The model under review builds one solid part; all positions refer to its coordinate system, in mm. Face numbers are marked on the shaded views. Coordinates: 2 decimals unless noted, no trailing zeros. Order: outer loops, then holes, each group sorted by start corner. A loop starts at its lowest first (then second) coordinate and runs counter-clockwise, first axis right, second up. Notation, with made-up numbers: (-10.5, 82) -> (44.5, 82) arc R18 cw to (44.5, 91) -> close; hole circle Ø2 at (85, 36). An arc over 180 degrees is marked (long way). Use one line per item in the form item = value. Start each with the question number.
(1) Take a section at B-B (z = -15). State the section outline as (x, y) points, then the cut area to 3 significant figures.
(2) Mouldability with a two-part tool opening along X and no side actions: class the marked faces 1, 2 and 3 as +X half, -X half, draft (parallel to the pull), parting line (faces both ways), or undercut.
(3) Insertion check: pin 1 Ø2.5 at (x, z) = (-36.2, -39.2) entering from -Y. The pin has a flat end and moves straight along its axis. Give the tip position at first contact, or say it passes through.
(4) Wall thickness on line 1 along X through (y, z) = (2, -21.5); line 2 along Z through (x, y) = (-81, 6.5); line 3 along X through (y, z) = (4, -3): over which ranges is each line inside the solid? List them lowest first.
(5) Take a section at D-D (z = -32.5). State the section outline as (x, y) points.
(6) Take a section at C-C (x = -36). State the section outline as (y, z) points.
(7) Take a section at A-A (x = -21). State the section outline as (y, z) points.
```python
from build123d import *

# Parameters (mm, degrees)
SKETCH1_W             = 115
SKETCH1_H             = 45
BOSS_EXTRUDE1_DEPTH   = 25
SKETCH2_R             = 11.7
SKETCH2_R_2           = 16.9
CUT_EXTRUDE1_DEPTH    = 26
M5X0_8_TAPPED_HOLE1_D = 4.2
M4X0_7_TAPPED_HOLE1_D = 3.3


with BuildPart() as part:
    # Sketch1 → Boss-Extrude1 (new body)
    with BuildSketch(Plane(origin=(0, 0, 0), x_dir=(1, 0, 0), z_dir=(0, 1, 0))):
        with Locations((-57.5, 22.5)):
            Rectangle(SKETCH1_W, SKETCH1_H)
    extrude(amount=BOSS_EXTRUDE1_DEPTH)

    # Sketch2 → Cut-Extrude1 (cut, through all)
    with BuildSketch(Plane.XZ):
        with Locations((-81, -15)):
            Circle(SKETCH2_R)
        with Locations((-21, -24)):
            Circle(SKETCH2_R_2)
    extrude(amount=-CUT_EXTRUDE1_DEPTH, mode=Mode.SUBTRACT)

    # M5x0.8 Tapped Hole1 (through all)
    with Locations(Plane(origin=(0, 0, 0), x_dir=(-1, 0, 0), z_dir=(0, -1, 0))):
        with Locations((36.202795796, 39.202795796), (5.797204204, 39.202795796), (5.797204204, 8.797204204), (36.202795796, 8.797204204)):
            Hole(M5X0_8_TAPPED_HOLE1_D / 2)

    # M4x0.7 Tapped Hole1 (through all)
    with Locations(Plane(origin=(0, 0, 0), x_dir=(-1, 0, 0), z_dir=(0, -1, 0))):
        with Locations((92.313708499, 3.686291501), (97, 15), (92.313708499, 26.313708499), (69.686291501, 26.313708499), (65, 15), (69.686291501, 3.686291501)):
            Hole(M4X0_7_TAPPED_HOLE1_D / 2)


solid = part.part
```
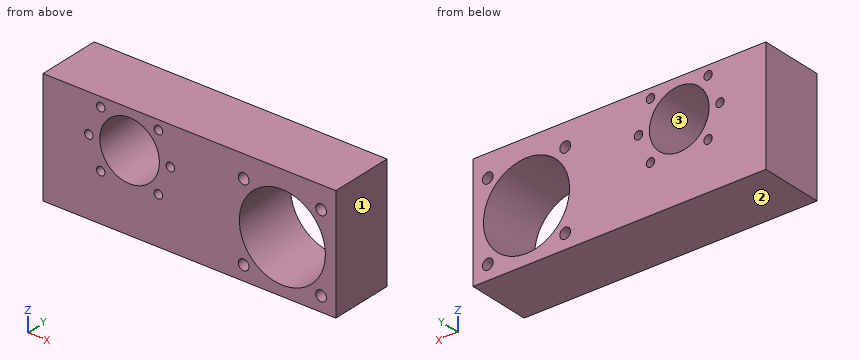
Findings:
q1.outline = (-115, 0) -> (-98.65, 0) -> (-98.65, 25) -> (-115, 25) -> close; (-95.35, 0) -> (-92.7, 0) -> (-92.7, 25) -> (-95.35, 25) -> close; (-69.3, 0) -> (-66.65, 0) -> (-66.65, 25) -> (-69.3, 25) -> close; (-63.35, 0) -> (-35.3, 0) -> (-35.3, 25) -> (-63.35, 25) -> close; (-6.7, 0) -> (0, 0) -> (0, 25) -> (-6.7, 25) -> close
q1.area = 1,410 mm²
q2.face_1 = +X half
q2.face_2 = draft
q2.face_3 = undercut
q3.pin_1 = through
q4.line_1 = -115 to -90.73, -71.27 to -37.71, -4.29 to 0
q4.line_2 = -45 to -26.7, -3.3 to 0
q4.line_3 = -115 to -93.81, -90.81 to -71.19, -68.19 to 0
q5.outline = (-115, 0) -> (-35.61, 0) -> (-35.61, 25) -> (-115, 25) -> close; (-6.39, 0) -> (0, 0) -> (0, 25) -> (-6.39, 25) -> close
q6.outline = (0, -45) -> (25, -45) -> (25, -41.29) -> (0, -41.29) -> close; (0, -37.11) -> (25, -37.11) -> (25, -31.79) -> (0, -31.79) -> close; (0, -16.21) -> (25, -16.21) -> (25, -10.89) -> (0, -10.89) -> close; (0, -6.71) -> (25, -6.71) -> (25, 0) -> (0, 0) -> close
q7.outline = (0, -45) -> (25, -45) -> (25, -40.9) -> (0, -40.9) -> close; (0, -7.1) -> (25, -7.1) -> (25, 0) -> (0, 0) -> close
